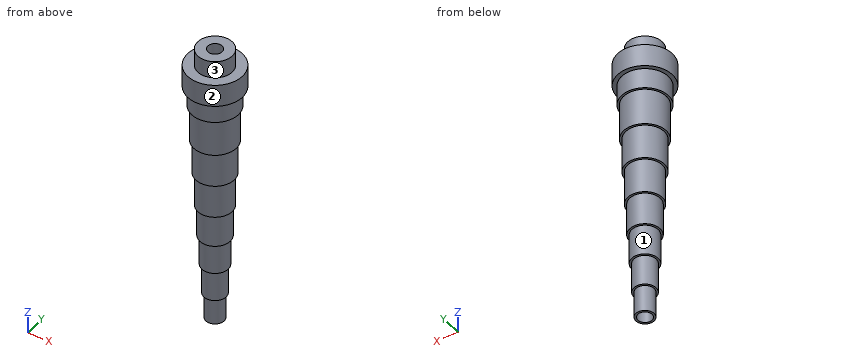
from build123d import *


with BuildPart() as part:
    # Sketch1 → Revolve1 (revolve)
    with BuildSketch(Plane(origin=(0, 0, 0), x_dir=(0, 0, -1), z_dir=(1, 0, 0)), mode=Mode.PRIVATE) as revolve1_sk:
        Polygon((-264.03808, 12.7), (213.40064, 12.7), (213.40064, 16.31696), (166.38016, 16.31696), (166.38016, 19.93392), (112.12576, 19.93392), (112.12576, 23.55088), (57.87136, 23.55088), (57.87136, 27.16784), (0, 27.16784), (0, 30.7848), (-61.48832, 30.7848), (-61.48832, 34.40176), (-122.97664, 34.40176), (-122.97664, 38.01872), (-188.08192, 38.01872), (-188.08192, 41.63568), (-224.25152, 41.63568), (-224.25152, 48.8696), (-264.03808, 48.8696), (-264.03808, 38.01872), (-264.03808, 30.7848), (-294.51808, 30.7848), (-294.51808, 12.7), align=None)
    revolve(revolve1_sk.sketch.rotate(Axis((0, 0, 19.904928919), (0, 0, -1)), 90), axis=Axis((0, 0, 19.904928919), (0, 0, -1)))


solid = part.part
Part model, mm, in its own coordinate system. Face numbers are marked on the shaded views. A direction names the side the tool comes from. Coordinates: 2 decimals unless noted, no trailing zeros. Loops run counter-clockwise (first coordinate to the right, second up) from the corner with the lowest first, then second, coordinate; pieces in that order, holes last. Notation, with made-up numbers: (64.5, 17) -> (81.5, 17) arc R28 ccw to (81.5, 48) -> close; hole circle Ø6 at (16.5, 41). An arc over 180 degrees is marked (long way). Use a Markdown table: item, result. Add a question column.
Item 1: Which spindle directions (+Z, -Z, +X, -X, +Y, -Y) get a long thin tool onto all of the face, cutting with end or side? Do the marked faces 1, 2 and 3. Say none if no direction does.
Item 2: Probe probe 1 along Y at (x, z) = (0, -57.5); probe 2 along Y at (x, z) = (0, -65); probe 3 along Z at (x, y) = (-11, 25.5). List the from-to ranges inside material, lowest first.
Item 3: Band-saw the part on A-A on z = -75. Write the cut outline in (x, y), plus the area to 3 significant figures.
Item 4: Flat gauge pins, fed straight in: P1, Ø1, axis at y = 6.5, z = 89.5, coming from the -X side; P2, Ø5, axis at x = -34, y = 32, coming from the +Z side; P3, Ø10, axis at y = 10, z = -120, coming from the -X side. Where does each tip first touch, or does it go through?
Geometry says:
| question | item | result |
|---|---|---|
| 1 | face 1 | -Z |
| 1 | face 2 | +Z, -Z |
| 1 | face 3 | +Z |
| 2 | probe 1 | -27.17 to -12.7, 12.7 to 27.17 |
| 2 | probe 2 | -23.55 to -12.7, 12.7 to 23.55 |
| 2 | probe 3 | 0 to 294.52 |
| 3 | outline | circle Ø47.1 at (0, 0); hole circle Ø25.4 at (0, 0) |
| 3 | area | 1,240 mm² |
| 4 | P1 | x = -33.87 |
| 4 | P2 | z = 264.04 |
| 4 | P3 | x = -19.3 |
